```python
from build123d import *

# Parameters (mm, degrees)
F1_DEPTH      = 5
F4_R          = 1.8
F5_DEPTH      = 25
F4_R_2        = 3.3576804347
F6_DEPTH      = 5
F6_DEPTH_BACK = 5.36


with BuildPart() as f1:
    # F0 (on Front) → F1 (new body)
    with BuildSketch(Plane.XZ):
        with BuildLine():
            ThreePointArc((-4, 0), (0, 4), (4, 0))
            Line((4, 0), (4, 11.2083284184))
            Line((4, 11.2083284184), (-4, 11.2083284184))
            Line((-4, 11.2083284184), (-4, 0))
        make_face()
        with BuildLine():
            Line((4, 0), (2.75, 0))
            ThreePointArc((2.75, 0), (0, -2.75), (-2.75, 0))
            Line((-2.75, 0), (-4, 0))
            ThreePointArc((-4, 0), (0, -4), (4, 0))
        make_face()
        with BuildLine():
            ThreePointArc((-2.75, 0), (0, 2.75), (2.75, 0))
            Line((2.75, 0), (4, 0))
            ThreePointArc((4, 0), (0, 4), (-4, 0))
            Line((-4, 0), (-2.75, 0))
        make_face()
    extrude(amount=F1_DEPTH)

    # F4 (on face) → F5 (cut)
    with BuildSketch(Plane(origin=(2.7526911935, 2.7526911935, 0), x_dir=(-0.7071067812, 0.7071067812, 0), z_dir=(0.7071067812, 0.7071067812, 0))):
        with Locations((-1.8839619588, 6.8741668947)):
            Circle(F4_R)
    extrude(amount=-F5_DEPTH, mode=Mode.SUBTRACT)

    # F4 (on face) → F6 (join, two sides)
    with BuildSketch(Plane(origin=(2.7526911935, 2.7526911935, 0), x_dir=(-0.7071067812, 0.7071067812, 0), z_dir=(0.7071067812, 0.7071067812, 0))) as f6_sk:
        with Locations((-1.8839619588, 6.8741668947)):
            Circle(F4_R_2)
        with Locations((-1.8839619588, 6.8741668947)):
            Circle(F4_R, mode=Mode.SUBTRACT)
    extrude(amount=F6_DEPTH)
    extrude(f6_sk.sketch, amount=-F6_DEPTH_BACK)


solid = f1.part
```
Design review of the part built by this model. Coordinates are the model's own, in mm. Coordinates: 2 decimals unless noted, no trailing zeros. Loops run counter-clockwise (first coordinate to the right, second up) from the corner with the lowest first, then second, coordinate; pieces in that order, holes last. Notation, with made-up numbers: (-27, -20.75) -> (-4, -20.75) arc R22 cw to (-4, -10.75) -> close; hole circle Ø9 at (-32.5, 33). An arc over 180 degrees is marked (long way). Answer as a JSON object with one key per item and string values.
Q1. Take a section at C-C on y = -3. Give the number of separate pieces and of enclosed holes in the cut face, plus the area to 3 significant figures.
Answer block:
{"separate pieces": "1", "enclosed holes": "2", "area": "77.4 mm^2"}
Q2. Clearance check with flat-ended pins moving along their axes: pin 1 Ø4 at (x, y) = (7.5, 4) entering from -Z; pin 2 Ø1.5 at (y, z) = (0, 8.5) entering from +X; pin 3 Ø5 at (x, z) = (1, 4) entering from +Y. State where each tip first meets the part, or that it passes through.
Answer block:
{"pin 1": "stops at z = 3.52", "pin 2": "stops at x = 7.72", "pin 3": "stops at y = 4.67"}
Q3. To check wall thickness, follow L1, parallel to Z at x = 0, y = -2.5; L2, parallel to Z at x = 1.75, y = -2; L3, parallel to Y at x = -3, z = 10.5. State the ranges of each line that lie inside material, in increasing order.
Answer block:
{"L1": "z = -4 to -2.75, 2.75 to 5.08, 8.67 to 11.21", "L2": "z = -3.6 to -2.12, 2.12 to 5.25, 8.5 to 11.21", "L3": "y = -5 to 0"}
Q4. The part is to be moulded in two halves that separate along Z. For faces 1 (the cylindrical face through (2.558, 4.423, 7.883)), 2 (the flat face through (4, -3, 4)), 3 (the cylindrical face through (-0.596, -2.465, 2.685)), say which applies: +Z half, -Z half, draft (parallel to the pull), parting line (faces both ways), or undercut.
Answer block:
{"face 1": "parting line", "face 2": "draft", "face 3": "undercut"}
Q5. Take a section at B-B on z = 9.75. Give the boundary of the cut face in (x, y).
Answer block:
{"outline": "(-4, -5) -> (4, -5) -> (4, -1.12) -> (8.85, 3.73) -> (6.39, 6.18) -> (0.21, 0) -> (-4, 0) -> close"}
Q6. Take a section at A-A on z = -0.25. Give the boundary of the cut face in (x, y).
Answer block:
{"outline": "(-3.99, -5) -> (-2.74, -5) -> (-2.74, 0) -> (-3.99, 0) -> close; (2.74, -5) -> (3.99, -5) -> (3.99, 0) -> (2.74, 0) -> close"}
Q7. Take a section at D-D on z = -2.5. Give the boundary of the cut face in (x, y).
Answer block:
{"outline": "(-3.12, -5) -> (-1.15, -5) -> (-1.15, 0) -> (-3.12, 0) -> close; (1.15, -5) -> (3.12, -5) -> (3.12, 0) -> (1.15, 0) -> close"}
